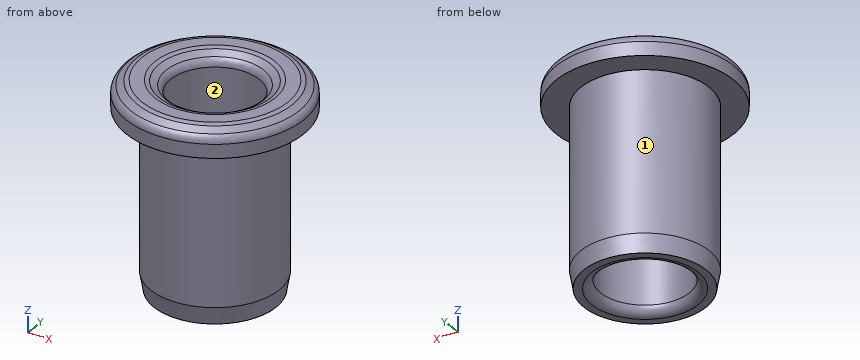
```python
from build123d import *

# Parameters (mm, degrees)
F0_R     = 18.415
F1_DEPTH = 50.8
F2_R     = 25.4
F2_R_2   = 18.415
F3_DEPTH = 7.62
F4_R     = 12.7
F5_DEPTH = 58.421
F6_SIZE2 = 2.1997045256
F6_SIZE  = 3.81
F7_R     = 2.54
F8_R     = 2.54
F9_SIZE2 = 0.895741062
F9_SIZE  = 5.08


with BuildPart() as f1:
    # F0 (on Top) → F1 (new body)
    with BuildSketch(Plane.XY):
        Circle(F0_R)
    extrude(amount=F1_DEPTH)

    # F2 (on face) → F3 (join)
    with BuildSketch(Plane.XY.offset(50.8)):
        Circle(F2_R)
        Circle(F2_R_2, mode=Mode.SUBTRACT)
        Circle(F2_R_2)
    extrude(amount=F3_DEPTH)

    # F4 (on face) → F5 (cut, through all)
    with BuildSketch(Plane.XY.offset(58.42)):
        Circle(F4_R)
    extrude(amount=-F5_DEPTH, mode=Mode.SUBTRACT)

    # F6
    f6_edges = [f1.edges().sort_by_distance(p)[0] for p in [
        (-25.4, 0, 58.42),
        (-12.7, 0, 58.42),
    ]]
    f6_side = f1.faces().sort_by_distance((-24.68158, 0, 58.42))[0]
    chamfer(f6_edges, length=F6_SIZE, length2=F6_SIZE2, reference=f6_side)

    # F7
    f7_edges = [f1.edges().sort_by_distance(p)[0] for p in [
        (-16.51, 0, 58.42),
        (-21.59, 0, 58.42),
        (-25.4, 0, 56.220295),
        (-12.7, 0, 56.220295),
    ]]
    fillet(f7_edges, radius=F7_R)

    # F8
    f8_edges = [f1.edges().sort_by_distance(p)[0] for p in [
        (-12.7, 0, 0),
    ]]
    fillet(f8_edges, radius=F8_R)

    # F9
    f9_edges = [f1.edges().sort_by_distance(p)[0] for p in [
        (-18.415, 0, 0),
    ]]
    f9_side = f1.faces().sort_by_distance((-18.415, 0, 25.4))[0]
    chamfer(f9_edges, length=F9_SIZE, length2=F9_SIZE2, reference=f9_side)


solid = f1.part
```
Source: CAD feature listing. Evaluate the final solid. Frame: model axes, mm. Face numbers are marked on the shaded views. A direction names the side the tool comes from. Coordinates: 2 decimals unless noted, no trailing zeros. Write each loop counter-clockwise with the first axis right and the second up, starting at its lowest first coordinate (ties: lowest second). Pieces come first, ordered by that corner, then holes. Notation, with made-up numbers: (65, 1.5) -> (102, 1.5) arc R35 ccw to (102, 34.5) -> close; hole circle Ø10 at (70, 73). An arc over 180 degrees is marked (long way). Return JSON: item names as keys, results as strings. Group by question number.
1) Contact query for flat-ended pins moving along their axis: P1, Ø8, axis at x = 20, y = 9, coming from the +Z side; P2, Ø12, axis at x = -17.5, z = 24, coming from the -Y side; P3, Ø12, axis at y = -18, z = 42.5, coming from the -X side; P4, Ø12, axis at x = 4.5, z = 14.5, coming from the -Y side (3 decimals). Output: stop coordinate, or through.
2) Ray query, line 1 along Y through (x, z) = (0, 17) (3 decimals); line 2 along Z through (x, y) = (-6.5, -20); line 3 along X through (y, z) = (2, 48.5). Return the intervals inside material, ascending.
3) Set-up query: the marked faces 1 and 2. Return all of +Z, -Z, +X, -X, +Y, -Y with unobstructed straight access to the full face (end or side cutting, diameter ignored); none if empty.
4) Section query A-A, the plane z = 32.5. Return loops of the section in (x, y) (3 decimals), plus the area to 3 significant figures.
From the geometry:
{
 "1": {"P1": "z = 58.42", "P2": "y = -14.38", "P3": "x = -13.97", "P4": "y = -18.415"},
 "2": {"line 1": "-18.415 to -12.7, 12.7 to 18.415", "line 2": "50.8 to 58.42", "line 3": "-18.31 to -12.54, 12.54 to 18.31"},
 "3": {"face 1": "-Z", "face 2": "+Z, -Z"},
 "4": {"outline": "circle Ø36.83 at (0, 0); hole circle Ø25.4 at (0, 0)", "area": "559 mm²"}
}
